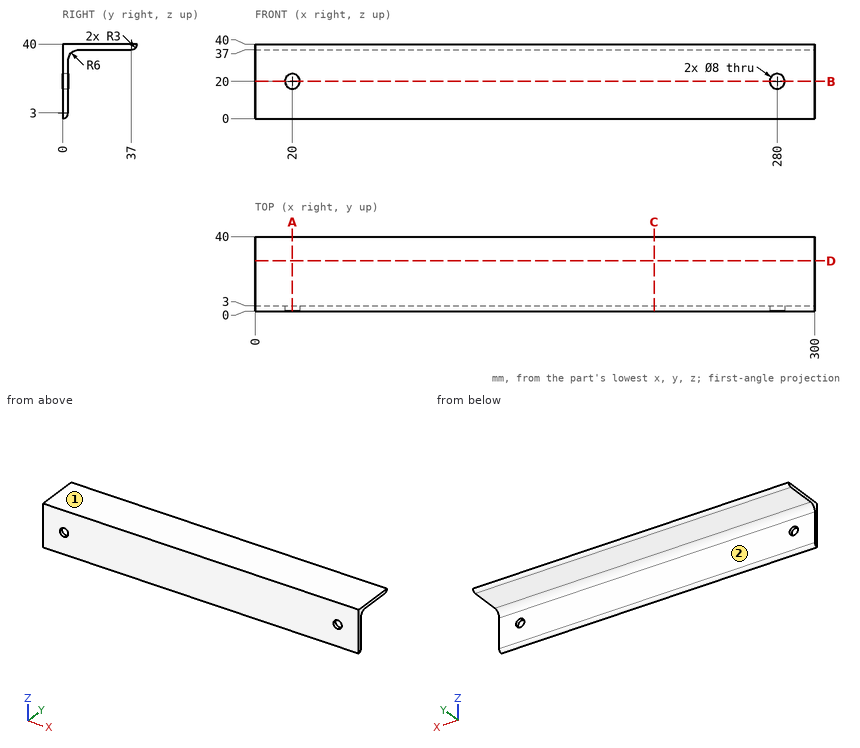
Geometry check sheet. Reference: drawing and pictorial views, mm from the part's lowest x, y, z. A direction names the side the tool comes from. Coordinates: 2 decimals unless noted, no trailing zeros. Write each loop counter-clockwise with the first axis right and the second up, starting at its lowest first coordinate (ties: lowest second). Pieces come first, ordered by that corner, then holes. Notation, with made-up numbers: (79, 51) -> (88, 51) arc R21 cw to (88, 82) -> close; hole circle Ø7 at (7.5, -16). An arc over 180 degrees is marked (long way). One line per question, with ' | ' between items.
1. Depth check by flat-ended pin: pin 1 Ø10 at (y, z) = (15.5, 31) entering from +X; pin 2 Ø6 at (x, z) = (76.5, 24) entering from -Y; pin 3 Ø8.5 at (x, z) = (85.5, 23.5) entering from +Y. Enter the tip coordinate at first touch or a pass-through.
Answers:
pin 1: passes through | pin 2: stops at y = 0 | pin 3: stops at y = 3
2. Cross-section at A-A on x = 20. Record the cut outline in (y, z).
Answers:
outline: (0, 0) arc R3 ccw to (3, 3) -> (3, 16) -> (0, 16) -> close; (0, 24) -> (3, 24) -> (3, 31) arc R6 cw to (9, 37) -> (37, 37) arc R3 ccw to (40, 40) -> (0, 40) -> close
3. Thickness scan on probe 1 along X at (y, z) = (2.35, 20); probe 2 along Z at (x, y) = (201.5, 34); probe 3 along Y at (x, z) = (173, 25). Record the ranges inside material, lowest first. Write a range as from..to.
Answers:
probe 1: x = 0..16, 24..276, 284..300 | probe 2: z = 37..40 | probe 3: y = 0..3
4. Set-up check for the marked faces 1 and 2: record each of +Z, -Z, +X, -X, +Y, -Y from which the full face is reachable in a straight line by a thin tool's end or side.
Answers:
face 1: +Z, +X, -X, +Y, -Y | face 2: -Z, +X, -X, +Y
5. Cross-section at D-D on y = 27. Record the cut outline in (x, z), and give its area (3 significant figures).
Answers:
outline: (0, 37) -> (300, 37) -> (300, 40) -> (0, 40) -> close | area: 900 mm²
6. Cross-section at B-B on z = 20. Record the cut outline in (x, y), and give its area (3 significant figures).
Answers:
outline: (0, 0) -> (16, 0) -> (16, 3) -> (0, 3) -> close; (24, 0) -> (276, 0) -> (276, 3) -> (24, 3) -> close; (284, 0) -> (300, 0) -> (300, 3) -> (284, 3) -> close | area: 852 mm²
7. Cross-section at C-C on x = 214. Record the cut outline in (y, z), and give its area (3 significant figures).
Answers:
outline: (0, 0) arc R3 ccw to (3, 3) -> (3, 31) arc R6 cw to (9, 37) -> (37, 37) arc R3 ccw to (40, 40) -> (0, 40) -> close | area: 235 mm²
